```python
from build123d import *

# Parameters (mm, degrees)
SKETCH_1_W                = 50
SKETCH_1_H                = 3
BLOCKEXTRUDE_DEPTH        = 50
FILLET_2_R                = 3
SKETCH_2_R                = 7.1
COAXIAL_FEEDTHROUGH_DEPTH = 71.774289117


with BuildPart() as part:
    # 草图1 → BlockExtrude (new body)
    with BuildSketch(Plane.XY):
        with Locations((25, 1.5)):
            Rectangle(SKETCH_1_W, SKETCH_1_H)
    extrude(amount=BLOCKEXTRUDE_DEPTH)

    # Fillet 2
    fillet_2_edges = [part.edges().sort_by_distance(p)[0] for p in [
        (50, 1.5, 50),
        (0, 1.5, 50),
        (50, 1.5, 0),
        (0, 1.5, 0),
    ]]
    fillet(fillet_2_edges, radius=FILLET_2_R)

    # 草图2 → Coaxial_feedthrough (cut, through all)
    with BuildSketch(Plane(origin=(0, 3, 0), x_dir=(1, 0, 0), z_dir=(0, 1, 0))):
        with Locations(Location((25, -25, 0), (0, 0, 270))):
            Circle(SKETCH_2_R)
    extrude(amount=-COAXIAL_FEEDTHROUGH_DEPTH, mode=Mode.SUBTRACT)


solid = part.part
```
Work out the finished part from the listing and answer in its coordinate system (mm). Coordinates: 2 decimals unless noted, no trailing zeros. Loops run counter-clockwise (first coordinate to the right, second up) from the corner with the lowest first, then second, coordinate; pieces in that order, holes last. Notation, with made-up numbers: (42, -6.5) - (101, -6.5) arc R8 cw to (101, -1.5) - close; hole circle Ø8 at (11, 9). An arc over 180 degrees is marked (long way). Use a Markdown table: item, result.
Item 1: Find section C-C, the plane y = 0.6. Determine the outline of the cut face in (x, z).
Evaluation:
| item | result |
|---|---|
| outline | (0, 3) arc R3 ccw to (3, 0) - (47, 0) arc R3 ccw to (50, 3) - (50, 47) arc R3 ccw to (47, 50) - (3, 50) arc R3 ccw to (0, 47) - close; hole circle Ø14.2 at (25, 25) |
Item 2: Consider probe 1 along X at (y, z) = (2, 25); probe 2 along X at (y, z) = (2.45, 24). Determine where each line is inside the solid, lowest interval first. Write a range as from..to.
Evaluation:
| item | result |
|---|---|
| probe 1 | x = 0..17.9, 32.1..50 |
| probe 2 | x = 0..17.97, 32.03..50 |
Item 3: Find section B-B, the plane x = 25. Determine the outline of the cut face in (y, z), and give its area (3 significant figures).
Evaluation:
| item | result |
|---|---|
| outline | (0, 0) - (3, 0) - (3, 17.9) - (0, 17.9) - close; (0, 32.1) - (3, 32.1) - (3, 50) - (0, 50) - close |
| area | 107 mm2 |
Item 4: Given pin 1 Ø13 at (x, z) = (25, 25) entering from -Y, flat-ended and moving along its own axis, determine where the tip first touches the part or whether it passes through.
Evaluation:
| item | result |
|---|---|
| pin 1 | passes through |
Item 5: The mould has two halves that part along Z. Classify faces 1 (the cylindrical face through (27.133, 1.521, 31.772)), 2 (the flat face through (0, 1, 25)), 3 (the flat face through (25, 2, 0)): +Z half, -Z half, draft (parallel to the pull), parting line (faces both ways), or undercut.
Evaluation:
| item | result |
|---|---|
| face 1 | undercut |
| face 2 | draft |
| face 3 | -Z half |
Item 6: Find section A-A, the plane z = 25. Determine the outline of the cut face in (x, y).
Evaluation:
| item | result |
|---|---|
| outline | (0, 0) - (17.9, 0) - (17.9, 3) - (0, 3) - close; (32.1, 0) - (50, 0) - (50, 3) - (32.1, 3) - close |
